from build123d import *

# Parameters (mm, degrees)
F0_W     = 114.545062
F0_H     = 134.937272
F0_W_2   = 34.949101
F0_H_2   = 32.08442
F1_DEPTH = 25.4


with BuildPart() as f1:
    # F0 (on Top) → F1 (new body)
    with BuildSketch(Plane.XY):
        Rectangle(F0_W, F0_H)
        with Locations((-24.042237, -35.384219)):
            Rectangle(F0_W_2, F0_H_2, mode=Mode.SUBTRACT)
        Polygon((33.824306, -53.145237), (2.885755, -53.145237), (2.885755, 6.695721), (-46.111111, 6.695721), (-46.111111, 34.831312), (51.882621, 34.831312), (51.882621, 6.695721), (33.824306, 6.695721), align=None, mode=Mode.SUBTRACT)
    extrude(amount=F1_DEPTH)


solid = f1.part
The listing builds one solid part. Answer for the finished solid, in the listing's coordinates (mm). A direction names the side the tool comes from. Round coordinates to 2 decimals unless told otherwise and drop trailing zeros. Order: outer loops, then holes, each group sorted by start corner. A loop starts at its lowest first (then second) coordinate and runs counter-clockwise, first axis right, second up. Notation, with made-up numbers: (77.25, -30) -> (99.25, -30) arc R21 cw to (99.25, -20) -> close; hole circle Ø10 at (63.25, -32). An arc over 180 degrees is marked (long way). One line per item, written item: value.
Item 1: For faces 5 (the flat face through (51.883, 21, 13)), 6 (the flat face through (-1, 67.469, 13)), determine the directions among +Z, -Z, +X, -X, +Y, -Y from which every point of the face is accessible in a straight line to the end or side of a thin tool.
Taken from the geometry:
face 5: +Z, -Z
face 6: +Z, -Z, +X, -X, +Y
Item 2: Find section D-D, the plane x = -1. Give the vertices of the cut face in (y, z).
Taken from the geometry:
outline: (-67.47, 0) -> (6.7, 0) -> (6.7, 25.4) -> (-67.47, 25.4) -> close; (34.83, 0) -> (67.47, 0) -> (67.47, 25.4) -> (34.83, 25.4) -> close
Item 3: Find section A-A, the plane x = -38. Give the vertices of the cut face in (y, z).
Taken from the geometry:
outline: (-67.47, 0) -> (-51.43, 0) -> (-51.43, 25.4) -> (-67.47, 25.4) -> close; (-19.34, 0) -> (6.7, 0) -> (6.7, 25.4) -> (-19.34, 25.4) -> close; (34.83, 0) -> (67.47, 0) -> (67.47, 25.4) -> (34.83, 25.4) -> close
Item 4: Straight lines are drawn through the part: L1, parallel to Y at x = -26, z = 23.25; L2, parallel to X at y = -41, z = 4.25; L3, parallel to X at y = 12, z = 16.75. For each, find the intervals that lie inside material, in ascending order.
Taken from the geometry:
L1: y = -67.47 to -51.43, -19.34 to 6.7, 34.83 to 67.47
L2: x = -57.27 to -41.52, -6.57 to 2.89, 33.82 to 57.27
L3: x = -57.27 to -46.11, 51.88 to 57.27
Item 5: Find section C-C, the plane y = -42. Give the vertices of the cut face in (x, z), then the cut area to 3 significant figures.
Taken from the geometry:
outline: (-57.27, 0) -> (-41.52, 0) -> (-41.52, 25.4) -> (-57.27, 25.4) -> close; (-6.57, 0) -> (2.89, 0) -> (2.89, 25.4) -> (-6.57, 25.4) -> close; (33.82, 0) -> (57.27, 0) -> (57.27, 25.4) -> (33.82, 25.4) -> close
area: 1,240 mm2
Item 6: For a pull along X with two mould halves and no side action, classify faces 1 (the flat face through (19, -53.145, 13)), 2 (the flat face through (-24, -19.342, 13)), 3 (the flat face through (-1, 1, 0)), 4 (the flat face through (57.273, -1, 13)) as released by +X, released by -X, zero draft, split by the parting line, or undercut.
Taken from the geometry:
face 1: undercut
face 2: undercut
face 3: zero draft
face 4: released by +X
Item 7: Find section B-B, the plane z = 16.5. Give the vertices of the cut face in (x, y), then the cut area to 3 significant figures.
Taken from the geometry:
outline: (-57.27, -67.47) -> (57.27, -67.47) -> (57.27, 67.47) -> (-57.27, 67.47) -> close; hole (-46.11, 6.7) -> (2.89, 6.7) -> (2.89, -53.15) -> (33.82, -53.15) -> (33.82, 6.7) -> (51.88, 6.7) -> (51.88, 34.83) -> (-46.11, 34.83) -> close; hole (-41.52, -51.43) -> (-6.57, -51.43) -> (-6.57, -19.34) -> (-41.52, -19.34) -> close
area: 9,730 mm2
